For this review, take the finished solid that the model builds, in its own axes (mm). Face numbers are marked on the shaded views. A direction names the side the tool comes from. Give positions to 0.01 mm unless a question says otherwise; leave off trailing zeros. Write each loop counter-clockwise with the first axis right and the second up, starting at its lowest first coordinate (ties: lowest second). Pieces come first, ordered by that corner, then holes.
Q1. Mouldability with a two-part tool opening along X and no side actions: class the marked faces 1, 2, 3 and 4 as released by +X, released by -X, zero draft, split by the parting line, or undercut.
Q2. We need section D-D (z = 14). Write out the cut boundary in (x, y), then the cut area to 3 significant figures.
Q3. For line 1 (Y direction, x = -1, z = 26); line 2 (Y direction, x = -11.25, z = 23); line 3 (X direction, y = -6.25, z = 14), list the stretches that pass through material, from the lowest coordinate up.
Q4. Insertion check: P1, Ø1, axis at y = -9, z = 26.5, coming from the +X side; P2, Ø1.5, axis at y = -3, z = 11, coming from the +X side; P3, Ø0.5, axis at x = -0.5, z = 24.5, coming from the -Y side. Each pin has a flat end and moves straight along its axis. Give the tip position at first contact, or say it passes through.
Q5. Machinability: for the marked faces 5 and 6, which of the approach directions +Z, -Z, +X, -X, +Y, -Y give a long, thin tool a straight path to every point of the face, cutting with its end or side? Answer none if there is none.
Q6. We need section C-C (y = -1.25). Write out the cut boundary in (x, z).
Q7. We need section B-B (x = -8.75). Write out the cut boundary in (y, z).
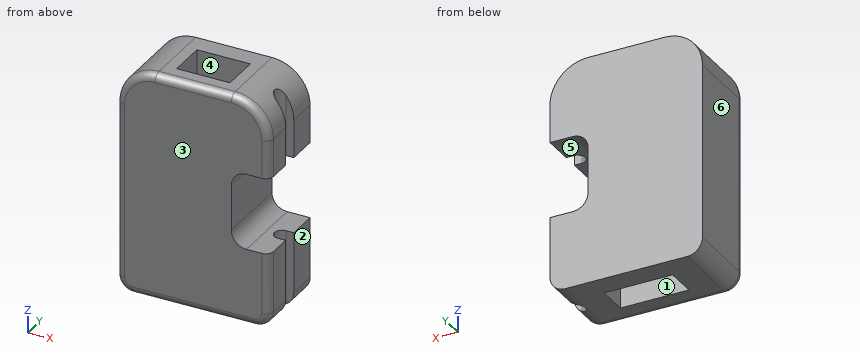
```python
from build123d import *

# Parameters (mm, degrees)
F1_DEPTH  = 10
F2_R      = 1
F3_W      = 2
F3_H      = 2
F4_DEPTH  = 20
F5_R      = 2
F6_R      = 2
F7_W      = 7
F7_H      = 5
F8_DEPTH  = 8
F9_R      = 0.99999
F10_W     = 9
F10_H     = 4
F11_DEPTH = 6


# Not quite as in the source:
# - a fillet or chamfer is up to 0.001 mm smaller than in the source, because OpenCascade refuses the exact size


with BuildPart() as f1:
    # F0 (on Front) → F1 (new body)
    with BuildSketch(Plane.XZ):
        with BuildLine():
            Line((-18, 0), (-2, 0))
            ThreePointArc((-2, 0), (-0.5857864376, 0.5857864376), (0, 2))
            Line((0, 2), (0, 10))
            Line((0, 10), (-5, 10))
            Line((-5, 10), (-5, 20))
            Line((-5, 20), (0, 20))
            Line((0, 20), (0, 25))
            ThreePointArc((0, 25), (-1.4644660941, 28.5355339059), (-5, 30))
            Line((-5, 30), (-15, 30))
            ThreePointArc((-15, 30), (-18.5355339059, 28.5355339059), (-20, 25))
            Line((-20, 25), (-20, 2))
            ThreePointArc((-20, 2), (-19.4142135624, 0.5857864376), (-18, 0))
        make_face()
    extrude(amount=F1_DEPTH)

    # F2
    f2_edges = [f1.edges().sort_by_distance(p)[0] for p in [
        (-10, -10, 30),
    ]]
    fillet(f2_edges, radius=F2_R)

    # F3 (on face) → F4 (cut, symmetric)
    with BuildSketch(Plane(origin=(0, 0, 20), x_dir=(1, 0, 0), z_dir=(0, 0, -1))):
        with Locations((-1, 5)):
            Rectangle(F3_W, F3_H)
    extrude(amount=F4_DEPTH, both=True, mode=Mode.SUBTRACT)

    # F5
    f5_edges = [f1.edges().sort_by_distance(p)[0] for p in [
        (-5, -5, 20),
    ]]
    fillet(f5_edges, radius=F5_R)

    # F6
    f6_edges = [f1.edges().sort_by_distance(p)[0] for p in [
        (-5, -5, 10),
    ]]
    fillet(f6_edges, radius=F6_R)

    # F7 (on face) → F8 (cut)
    with BuildSketch(Plane.XY.offset(30)):
        with Locations((-10, -5)):
            Rectangle(F7_W, F7_H)
    extrude(amount=-F8_DEPTH, mode=Mode.SUBTRACT)

    # F9 (radius 1 in the source; OpenCascade refuses exactly that, so slightly less here)
    f9_edges = [f1.edges().sort_by_distance(p)[0] for p in [
        (-2, -4, 24.5),
        (-2, -6, 24.5),
        (-2, -6, 5),
        (-2, -4, 5),
    ]]
    fillet(f9_edges, radius=F9_R)

    # F10 (on face) → F11 (cut)
    with BuildSketch(Plane(origin=(0, 0, 0), x_dir=(1, 0, 0), z_dir=(0, 0, -1))):
        with Locations((-10, 5)):
            Rectangle(F10_W, F10_H)
    extrude(amount=-F11_DEPTH, mode=Mode.SUBTRACT)


solid = f1.part
```
Computed:
1. face 1: undercut
1. face 2: released by +X
1. face 3: zero draft
1. face 4: undercut
2. outline: (-20, -9) arc R1 ccw to (-19, -10) - (-5, -10) - (-5, 0) - (-20, 0) - close
2. area: 150 mm2
3. line 1: y = -9.99 to -6, -4 to 0
3. line 2: y = -10 to -7.5, -2.5 to 0
3. line 3: x = -20 to -5
4. P1: stops at x = -0.1
4. P2: stops at x = -3.97
4. P3: stops at y = -9.97
5. face 5: +X, +Y, -Y
5. face 6: +Z, -Z, -X, +Y, -Y
6. outline: (-20, 2) arc R2 ccw to (-18, 0) - (-2, 0) arc R2 ccw to (0, 2) - (0, 10) - (-3, 10) arc R2 cw to (-5, 12) - (-5, 18) arc R2 cw to (-3, 20) - (0, 20) - (0, 25) arc R5 ccw to (-5, 30) - (-15, 30) arc R5 ccw to (-20, 25) - close
7. outline: (-10, 1) arc R1 ccw to (-9, 0) - (-7, 0) - (-7, 6) - (-3, 6) - (-3, 0) - (0, 0) - (0, 30) - (-2.5, 30) - (-2.5, 22) - (-7.5, 22) - (-7.5, 30) - (-9, 30) arc R1 ccw to (-10, 29) - close
